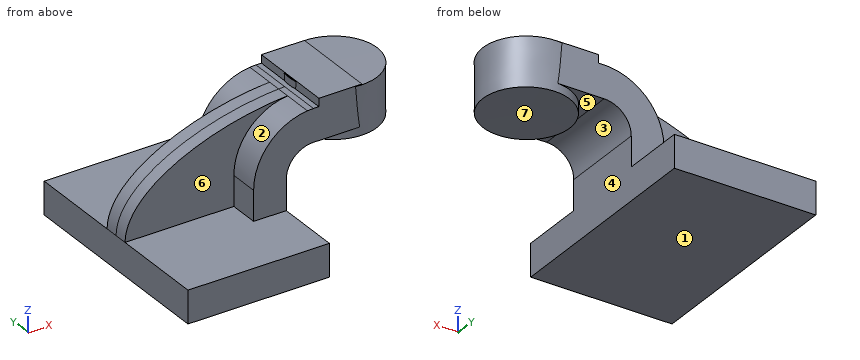
```python
from build123d import *

# Parameters (mm, degrees)
F1_DEPTH = 63.5
F2_DEPTH = 25.4
F3_DEPTH = 7.9375


with BuildPart() as f1:
    # F0 (on Front) → F1 (new body, symmetric)
    with BuildSketch(Plane.XZ):
        Polygon((22.225, 9.525), (-41.275, 9.525), (-41.275, -9.525), (41.275, -9.525), (41.275, 9.525), align=None)
    extrude(amount=F1_DEPTH, both=True)

    # F0 (on Front) → F2 (join, symmetric)
    with BuildSketch(Plane.XZ):
        with BuildLine():
            Line((22.225, 27.0002), (22.225, 9.525))
            Line((22.225, 9.525), (41.275, 9.525))
            Line((41.275, 9.525), (41.275, 27.0002))
            ThreePointArc((41.275, 27.0002), (45.9246798487, 38.2255201513), (57.15, 42.8752))
            Line((57.15, 42.8752), (60.325, 42.8752))
            Line((60.325, 42.8752), (60.325, 61.9252))
            Line((60.325, 61.9252), (57.15, 61.9252))
            add(Edge.make_bspline(
                [(53.6016861152, 61.7444814514), (54.7864461989, 61.817216834), (55.9695068539, 61.8775273392), (57.15, 61.9252)],
                knots=[108.7054668937, 108.7054668937, 108.7054668937, 108.7054668937, 111.5045361635, 111.5045361635, 111.5045361635, 111.5045361635], degree=3))
            ThreePointArc((53.6016861152, 61.7444814514), (31.2301187558, 50.4077923855), (22.225, 27.0002))
        make_face()
        Polygon((60.325, 66.675), (60.325, 61.9252), (60.325, 42.8752), (85.6790583176, 42.8752), (85.4500830173, 66.675), align=None)
    extrude(amount=F2_DEPTH, both=True)

    # F0 (on Front) → F3 (join, symmetric)
    with BuildSketch(Plane.XZ):
        with BuildLine():
            add(Edge.make_bspline(
                [(-41.275, 9.525), (-40.9848631129, 37.3550228275), (7.5899995014, 58.9197090153), (53.6016861152, 61.7444814514)],
                knots=[0, 0, 0, 0, 108.7054668937, 108.7054668937, 108.7054668937, 108.7054668937], degree=3))
            Line((-41.275, 9.525), (22.225, 9.525))
            Line((22.225, 9.525), (22.225, 27.0002))
            ThreePointArc((22.225, 27.0002), (31.2301187558, 50.4077923855), (53.6016861152, 61.7444814514))
        make_face()
    extrude(amount=F3_DEPTH, both=True)

    # F0 (on Front) → F4 (revolve)
    with BuildSketch(Plane.XZ):
        Polygon((85.4500830173, 66.675), (85.6790583176, 42.8752), (85.725, 38.1), (111.125, 38.1), (111.125, 66.675), align=None)
    revolve(axis=Axis((85.5875415087, 0, 52.3875), (-0.0096204465, 0, 0.9999537224)))


solid = f1.part
```
Here's how the part is built. I have some questions about the finished solid (model axes, mm). Face numbers are marked on the shaded views. A direction names the side the tool comes from. Round coordinates to 2 decimals unless told otherwise and drop trailing zeros. Order: outer loops, then holes, each group sorted by start corner. A loop starts at its lowest first (then second) coordinate and runs counter-clockwise, first axis right, second up. Notation, with made-up numbers: (4, 45) -> (44, 45) arc R29 cw to (44, 73) -> close; hole circle Ø7 at (-29.75, 63). An arc over 180 degrees is marked (long way). Use a Markdown table: item, result. Add a question column.
(1) For the marked faces 5, 6 and 7, which set-ups out of +Z, -Z, +X, -X, +Y, -Y let a thin tool reach every point of the face, with its end or its side?
(2) If we mould it in two halves opening along X, with no side actions, what happens to the marked faces 1, 2, 3 and 4? For each: released by +X, released by -X, zero draft, split by the parting line, or undercut.
(3) Suppose I cut it at A-A, the plane z = 6.5. Please give me the cut outline in (x, y) (3 decimals), and give its area (3 significant figures).
(4) Suppose I cut it at B-B, the plane y = 34. Please give me the cut outline in (x, z) (3 decimals).
(5) For pin 1 Ø19 at (y, z) = (19.5, 21) entering from -X (3 decimals); pin 2 Ø12 at (x, z) = (1, 16.5) entering from -Y; pin 3 Ø1 at (x, z) = (46, 40) entering from +Y; pin 4 Ø10 at (y, z) = (-42.5, 18.5) entering from -X, each with a flat end and sliding along its axis, tell me the tip position at first contact or that it passes through.
(6) I need wall thicknesses on line 1 along X through (y, z) = (20.5, 1.5) (3 decimals); line 2 along Y through (x, z) = (7, 33.5); line 3 along Z through (x, y) = (14, 32) (3 decimals). Which ranges of each line are inside material? Lowest first, please.
Verdict:
| question | item | result |
|---|---|---|
| 1 | face 5 | -Z |
| 1 | face 6 | +Z, -X, -Y |
| 1 | face 7 | -Z, +X |
| 2 | face 1 | zero draft |
| 2 | face 2 | released by -X |
| 2 | face 3 | undercut |
| 2 | face 4 | released by +X |
| 3 | outline | (-41.275, -63.5) -> (41.275, -63.5) -> (41.275, 63.5) -> (-41.275, 63.5) -> close |
| 3 | area | 10,500 mm2 |
| 4 | outline | (-41.275, -9.525) -> (41.275, -9.525) -> (41.275, 9.525) -> (-41.275, 9.525) -> close |
| 5 | pin 1 | x = 22.225 |
| 5 | pin 2 | y = -7.94 |
| 5 | pin 3 | y = 25.4 |
| 5 | pin 4 | through |
| 6 | line 1 | -41.275 to 41.275 |
| 6 | line 2 | -7.94 to 7.94 |
| 6 | line 3 | -9.525 to 9.525 |
